```python
from build123d import *

# Parameters (mm, degrees)
SKETCH1_R           = 2.8
BOSS_EXTRUDE1_DEPTH = 5
FILLET1_R           = 2
BOSS_EXTRUDE2_DEPTH = 6.4
FILLET2_R           = 2
SKETCH3_W           = 8
SKETCH3_H           = 2
CUT_EXTRUDE1_DEPTH  = 4
SKETCH6_W           = 104.287250585
SKETCH6_H           = 38
CUT_EXTRUDE3_DEPTH  = 5
FILLET3_R           = 2
BOSS_EXTRUDE3_DEPTH = 6.4
CUT_EXTRUDE4_DEPTH  = 52
FILLET4_R           = 20


with BuildPart() as part:
    # Sketch1 → Boss-Extrude1 (new body)
    with BuildSketch(Plane.XY):
        with BuildLine():
            Line((0, 19), (100, 19))
            ThreePointArc((100, 19), (111.005680352, 15.487898502), (117.942616866, 6.25))
            Line((117.942616866, 6.25), (87.942616866, 6.25))
            Line((87.942616866, 6.25), (87.942616866, -6.25))
            Line((87.942616866, -6.25), (117.942616866, -6.25))
            ThreePointArc((117.942616866, -6.25), (111.005680352, -15.487898502), (100, -19))
            Line((100, -19), (0, -19))
            ThreePointArc((0, -19), (-19, 0), (0, 19))
        make_face()
        Circle(SKETCH1_R, mode=Mode.SUBTRACT)
        with BuildLine():
            Line((29.217733251, 11), (59.217733251, 11))
            ThreePointArc((59.217733251, 11), (70.217733251, 0), (59.217733251, -11))
            Line((59.217733251, -11), (29.217733251, -11))
            ThreePointArc((29.217733251, -11), (18.217733251, 0), (29.217733251, 11))
        make_face(mode=Mode.SUBTRACT)
    extrude(amount=BOSS_EXTRUDE1_DEPTH)

    # Fillet1
    fillet1_edges = [part.edges().sort_by_distance(p)[0] for p in [
        (117.942616866, 6.25, 2.5),
        (117.942616866, -6.25, 2.5),
    ]]
    fillet(fillet1_edges, radius=FILLET1_R)

    # Sketch2 → Boss-Extrude2 (add)
    with BuildSketch(Plane.XY.offset(5)):
        with BuildLine():
            Line((73.942616866, 19), (73.942616866, -19))
            Line((73.942616866, -19), (100, -19))
            ThreePointArc((100, -19), (109.638693468, -16.373624774), (116.612668437, -9.220588235))
            ThreePointArc((116.612668437, -9.220588235), (116.587505946, -7.235400688), (114.863966496, -6.25))
            Line((114.863966496, -6.25), (87.942616866, -6.25))
            Line((87.942616866, -6.25), (87.942616866, 6.25))
            Line((87.942616866, 6.25), (114.863966496, 6.25))
            ThreePointArc((114.863966496, 6.25), (116.587505946, 7.235400688), (116.612668437, 9.220588235))
            ThreePointArc((116.612668437, 9.220588235), (109.638693468, 16.373624774), (100, 19))
            Line((100, 19), (73.942616866, 19))
        make_face()
    extrude(amount=BOSS_EXTRUDE2_DEPTH)

    # Fillet2
    fillet2_edges = [part.edges().sort_by_distance(p)[0] for p in [
        (73.942616866, 0, 5),
        (73.942616866, 0, 11.4),
    ]]
    fillet(fillet2_edges, radius=FILLET2_R)

    # Sketch3 → Cut-Extrude1 (cut)
    with BuildSketch(Plane.XY.offset(11.4)):
        with Locations((83.942616866, 0)):
            Rectangle(SKETCH3_W, SKETCH3_H)
    extrude(amount=-CUT_EXTRUDE1_DEPTH, mode=Mode.SUBTRACT)

    # Sketch6 → Cut-Extrude3 (cut)
    with BuildSketch(Plane(origin=(0, 0, 0), x_dir=(-1, 0, 0), z_dir=(0, 0, -1))):
        with Locations((-131.086242158, 0)):
            Rectangle(SKETCH6_W, SKETCH6_H)
    extrude(amount=-CUT_EXTRUDE3_DEPTH, mode=Mode.SUBTRACT)

    # Fillet3
    fillet3_edges = [part.edges().sort_by_distance(p)[0] for p in [
        (78.942616866, 0, 0),
        (78.942616866, 0, 5),
    ]]
    fillet(fillet3_edges, radius=FILLET3_R)

    # Sketch7 → Boss-Extrude3 (add)
    with BuildSketch(Plane.XY.offset(11.4)):
        with BuildLine():
            Line((114.863966496, 6.25), (110.942616866, 6.25))
            Line((110.942616866, 6.25), (110.942616866, -6.25))
            Line((110.942616866, -6.25), (114.863966496, -6.25))
            ThreePointArc((114.863966496, -6.25), (116.278180059, -6.835786438), (116.863966496, -8.25))
            Line((116.863966496, -8.25), (116.863966496, 8.25))
            ThreePointArc((116.863966496, 8.25), (116.278180059, 6.835786438), (114.863966496, 6.25))
        make_face()
    extrude(amount=-BOSS_EXTRUDE3_DEPTH)

    # Sketch8 → Cut-Extrude4 (cut)
    with BuildSketch(Plane.XY.offset(11.4)):
        Polygon((49.166460224, 20.686961638), (202.884451104, 0), (49.166460224, -20.686961638), (49.166460224, -34.841866296), (221.786697366, -38.976706561), (223.885725762, 48.652985565), (49.166460224, 52.838104681), (49.166460224, 51.155729305), align=None)
    extrude(amount=-CUT_EXTRUDE4_DEPTH, mode=Mode.SUBTRACT)

    # Fillet4
    fillet4_edges = [part.edges().sort_by_distance(p)[0] for p in [
        (61.701715921, -19, 2.5),
        (61.701715921, 19, 2.5),
    ]]
    fillet(fillet4_edges, radius=FILLET4_R)


solid = part.part
```
For this review, take the finished solid that the model builds, in its own axes (mm). A direction names the side the tool comes from. Round coordinates to 2 decimals unless told otherwise and drop trailing zeros. Write each loop counter-clockwise with the first axis right and the second up, starting at its lowest first coordinate (ties: lowest second). Pieces come first, ordered by that corner, then holes. Notation, with made-up numbers: (-6, 4) - (0, 4) arc R7 cw to (0, 15) - close; hole circle Ø6 at (57, 74.5). An arc over 180 degrees is marked (long way). Answer as a JSON object with one key per item and string values.
1. To check wall thickness, follow line 1 along Y through (x, z) = (0, 2.6); line 2 along Y through (x, z) = (45, 1); line 3 along X through (y, z) = (-6, 9.5). State the ranges of each line that lie inside material, in increasing order.
Response values:
{"line 1": "y = -19 to -2.8, 2.8 to 19", "line 2": "y = -19 to -11, 11 to 19", "line 3": "x = 73.95 to 87.94, 110.94 to 116.86"}
2. For pin 1 Ø1.9 at (x, z) = (99.5, 9.5) entering from +Y; pin 2 Ø2 at (x, y) = (4, -13.5) entering from +Z; pin 3 Ø1.2 at (x, z) = (82, 8.5) entering from +Y; pin 4 Ø3 at (x, y) = (96.5, -15) entering from +Z, all flat-tipped, find the tip position at first contact; note any pin that passes through.
Response values:
{"pin 1": "stops at y = 14.04", "pin 2": "stops at z = 5", "pin 3": "stops at y = 16.35", "pin 4": "stops at z = 11.4"}
3. Draft analysis for pull direction Y (two halves, no side actions). For faces 5 (the face through (116.864, 0, 8)), 6 (the face through (84, 1, 9)), 7 (the face through (-19, 0, 2)), 8 (the face through (44, -11, 2)), state which applies: +Y half, -Y half, draft (parallel to the pull), parting line (faces both ways), or undercut.
Response values:
{"face 5": "draft", "face 6": "undercut", "face 7": "parting line", "face 8": "undercut"}
4. Tool access review of faces 1 (the face through (87, -4, 11.4)), 2 (the face through (95, -7, 5)), 3 (the face through (73.943, 0, 8)), 4 (the face through (18.22, -0.24, 2.46)): name each direction out of +Z, -Z, +X, -X, +Y, -Y from which nothing blocks a thin tool from reaching the whole face with its end or side.
Response values:
{"face 1": "+Z, +X, -X, +Y, -Y", "face 2": "-Z, +X, +Y, -Y", "face 3": "+Z, -X, +Y, -Y", "face 4": "+Z, -Z"}
5. We need section A-A on x = 98.5. Give the boundary of the cut face in (y, z).
Response values:
{"outline": "(-14.05, 5) - (-6.25, 5) - (-6.25, 11.4) - (-14.05, 11.4) - close; (6.25, 5) - (14.05, 5) - (14.05, 11.4) - (6.25, 11.4) - close"}
6. We need section C-C on x = -10. Give the boundary of the cut face in (y, z), then the cut area to 3 significant figures.
Response values:
{"outline": "(-16.16, 0) - (16.16, 0) - (16.16, 5) - (-16.16, 5) - close", "area": "162 mm2"}
7. We need section B-B on y = 13. Give the boundary of the cut face in (x, z).
Response values:
{"outline": "(-13.86, 0) - (76.94, 0) arc R2 ccw to (78.94, 2) - (78.94, 3) arc R2 cw to (80.94, 5) - (106.29, 5) - (106.29, 11.4) - (75.94, 11.4) arc R2 ccw to (73.94, 9.4) - (73.94, 7) arc R2 cw to (71.94, 5) - (-13.86, 5) - close"}
